Geometry check sheet. Reference: the model listing, model coordinates, mm. A direction names the side the tool comes from. Coordinates: 2 decimals unless noted, no trailing zeros. Loops run counter-clockwise (first coordinate to the right, second up) from the corner with the lowest first, then second, coordinate; pieces in that order, holes last.
Autodesk Inventor part; units mm, degrees
ref_plane "Work Plane1" through (0, -20.15, 0) normal (-1, 0, 0) x (0, 0, 1)
ref_plane "YZ Plane" through (0, 0, 0) normal (1, 0, 0) x (0, 1, 0)
ref_plane "XZ Plane" through (0, 0, 0) normal (0, 1, 0) x (-1, 0, 0)
sketch "Sketch1" plane through (0, 0, 0) normal (0, 0, 1) x (1, 0, 0)
  line L0 (-12.05, 27.5) -> (12.05, 27.5)
  line L1 (12.05, 27.5) -> (12.05, -27.5)
  line L2 (12.05, -27.5) -> (-12.05, -27.5)
  line L3 (-12.05, -27.5) -> (-12.05, 27.5)
  line L4 (-10.05, 20.15) -> (10.05, 20.15)
  line L5 (10.05, 20.15) -> (10.05, -20.15)
  line L6 (10.05, -20.15) -> (-10.05, -20.15)
  line L7 (-10.05, -20.15) -> (-10.05, 20.15)
  line L8 (0, 0) -> (0, 17.7516) construction
  line L9 (0, 0) -> (17.0454, 0) construction
  line L10 (-12.05, -27.5) -> (12.05, -27.5)
  line L11 (12.05, -27.5) -> (12.05, -20.15)
  line L12 (12.05, -20.15) -> (-12.05, -20.15)
  line L13 (-12.05, -20.15) -> (-12.05, -27.5)
  circle A0 centre (-4.65, 24.5) radius 2.175
  circle A1 centre (4.65, 24.475) radius 2.175
  circle A2 centre (-4.6492, -24.5) radius 2.175
  circle A3 centre (4.65, -24.375) radius 2.175
  point P0 (12.05, -23.825)
  dimension "d0" = 40.3
  dimension "d1" = 20.1
  dimension "d2" = 55
  dimension "d3" = 24.1
  dimension "d4" = 4.35
  dimension "d5" = 4.325
  dimension "d6" = 4.35
  dimension "d8" = 4.35
  dimension "d9" = 5.4
  dimension "d13" = 5.4
  dimension "d28" = 48.85
  dimension "d29" = 9.3
  dimension "d30" = 9.3
extrude "Extrusion1" add sketch "Sketch1" along normal blind 5 contours L0 L1 L12 L5 L4 L7 L3 | L12 L6 L1 L2 L3
extrude "Extrusion2" add sketch "Sketch1" against normal blind 15 contours L12 L6 L1 L2 L3 | A2 | A3
extrude "Extrusion3" cut sketch "Sketch1" against normal blind 3 contours A2 | A3
sketch "Sketch2" plane through (-10.05, -20.15, 5) normal (0, 1, 0) x (1, 0, 0)
  circle A0 centre (5.9, 16) radius 1.05
  circle A1 centre (14.2, 16) radius 1.05
  line L0 (0, 0) -> (20.1, 0) construction
  line L1 (10.05, 0) -> (10.05, 23.167) construction
  line L2 (-2, 20) -> (22.1, 20)
  circle A2 centre (14.2, 16) radius 2
  circle A3 centre (5.9, 16) radius 2
  point P0 (10.05, 5)
  dimension "d20" = 2.1
  dimension "d21" = 8.3
  dimension "d22" = 4
  dimension "d23" = 4
extrude "Extrusion4" cut sketch "Sketch2" against normal blind 10 contours A0 | A1
extrude "Extrusion5" cut sketch "Sketch2" against normal blind 3 contours A0 | A1 | A2 | A3
sketch "Sketch3" plane through (12.05, -20.15, 0) normal (1, 0, 0) x (0, 0, -1)
  line L0 (0, 47.65) -> (-5, 47.65) construction
  line L1 (-5, 47.65) -> (38.6712, 47.65) construction
  line L2 (0, 0) -> (-5, 0) construction
  line L3 (-5, 0) -> (38.6712, 0) construction
  line L4 (0, 15) -> (15, 0)
  line L5 (0, 15) -> (0, 9.3431)
  line L6 (0, 9.3431) -> (9.3431, 0)
  line L7 (9.3431, 0) -> (15, 0)
  line L8 (15, 0) -> (15, -7.35) construction
  line L9 (15, -0.9137) -> (15, 2.4866) construction
  line L10 (-5, 0) -> (15, 0)
  line L11 (15, 0) -> (15, -15)
  line L12 (15, -15) -> (-5, -15)
  line L13 (-5, -15) -> (-5, 0)
  circle A0 centre (5, -12.35) radius 1.25
  line L14 (0, 0) -> (0, 47.65)
  line L15 (0, 47.65) -> (0, 0)
  line L16 (0, 0) -> (15, 0)
  line L17 (15, -7.35) -> (15, 0)
  line L18 (15, -7.35) -> (-5, -7.35)
  line L19 (-5, 47.65) -> (-5, -7.35)
  line L20 (0, 47.65) -> (-5, 47.65)
  point P0 (0, 20.15)
  dimension "d31" = 4
  dimension "d34" = 15
  dimension "d39" = 2.5
  dimension "d41" = 10
  dimension "d44" = 45
  dimension "d46" = 5
ref_plane "Work Plane1" through (0, -20.15, 0) normal (-1, 0, 0) x (0, 0, 1)
extrude "Extrusion6" add sketch "Sketch3" against normal up to surface (2 mm away) contours L4 L7 L6 L5
mirror "Mirror1" about plane through (0, -20.15, 0) normal (-1, 0, 0) of "Extrusion6"
extrude "Extrusion7" add sketch "Sketch3" along normal blind 3.9 from surface at -24.1 contours L11 L18 L13 L10 L7 | L11 L12 L13 L18 | A0
extrude "Extrusion8" cut sketch "Sketch3" against normal blind 35.65 contours A0
equation "\"d8\" = d6"
equation "\"d13\" = d9"
properties part number "BIGServoHolder"
1) Material ranges on probe 1 along X at (y, z) = (-21.8, -11); probe 2 along X at (y, z) = (-25.85, -11); probe 3 along Y at (x, z) = (4.65, 2), recorded low to high.
Data:
probe 1: x = -12.05 to -6.15, -2.15 to 2.15, 6.15 to 12.05
probe 2: x = -12.05 to -5.2, -3.1 to 3.1, 5.2 to 12.05
probe 3: y = -27.5 to -26.55, -22.2 to -20.15, 20.15 to 22.3, 26.65 to 27.5
2) Access from +Z, -Z, +X, -X, +Y, -Y to the whole of each face (thin tool, end or side, straight path). Record for faces 4 (the flat face through (2, -27.5, -5)), 5 (the flat face through (-11.064, -15.544, -4.737)), 6 (the flat face through (0, 20.15, 2)).
Data:
face 4: +Z, -Z, +X, -Y
face 5: +X, -X
face 6: +Z, -Z
3) Section check C-C on x = 4.15. Record the cut outline in (y, z).
Data:
outline: (-27.5, -15) - (-20.15, -15) - (-20.15, -13) - (-23.15, -13) - (-23.15, -12.05) - (-27.5, -12.05) - close; (-27.5, -9.95) - (-23.15, -9.95) - (-23.15, -9) - (-20.15, -9) - (-20.15, 5) - (-22.26, 5) - (-22.26, -3) - (-26.49, -3) - (-26.49, 5) - (-27.5, 5) - close; (20.15, 0) - (22.36, 0) - (22.36, 5) - (20.15, 5) - close; (26.59, 0) - (27.5, 0) - (27.5, 5) - (26.59, 5) - close
4) Mould release check, pull along X, two halves, no side actions. Record for faces 1 (the cylindrical face through (-10.073, -33.609, -5.577)), 2 (the flat face through (-8.15, -30, -5)), 3 (the flat face through (-3, -23.15, -10)): +X half, -X half, draft (parallel to the pull), parting line (faces both ways), or undercut.
Data:
face 1: draft
face 2: +X half
face 3: undercut
5) Depth check by flat-ended pin: pin 1 (2.5 mm diameter, centred on x = 4.15, z = -11, fed in from -Y); pin 2 (3 mm diameter, centred on x = -4.15, z = -11, fed in from +Y); pin 3 (1 mm diameter, centred on x = 10.5, y = -16.5, fed in from -Z). Enter the tip coordinate at first touch or a pass-through.
Data:
pin 1: stops at y = -27.5
pin 2: stops at y = -23.15
pin 3: stops at z = -11.85
6) Section check A-A on z = -11. Record the cut outline in (x, y).
Data:
outline: (-12.05, -35.15) - (-8.15, -35.15) - (-8.15, -27.5) - (-5.2, -27.5) - (-5.2, -23.15) - (-6.15, -23.15) - (-6.15, -20.15) - (-10.05, -20.15) - (-10.05, -16.15) - (-12.05, -16.15) - close; (-3.1, -27.5) - (3.1, -27.5) - (3.1, -23.15) - (2.15, -23.15) - (2.15, -20.15) - (-2.15, -20.15) - (-2.15, -23.15) - (-3.1, -23.15) - close; (5.2, -27.5) - (12.05, -27.5) - (12.05, -16.15) - (10.05, -16.15) - (10.05, -20.15) - (6.15, -20.15) - (6.15, -23.15) - (5.2, -23.15) - close
7) Section check D-D on z = -1.25. Record the cut outline in (x, y) (3 decimals).
Data:
outline: (-12.05, -35.15) - (-8.15, -35.15) - (-8.15, -27.5) - (12.05, -27.5) - (12.05, -20.15) - (-12.05, -20.15) - close; (-12.05, -12.057) - (-10.05, -12.057) - (-10.05, -6.4) - (-12.05, -6.4) - close; (10.05, -12.057) - (12.05, -12.057) - (12.05, -6.4) - (10.05, -6.4) - close; hole circle Ø4.35 at (-4.649, -24.5); hole circle Ø4.35 at (4.65, -24.375)
8) Section check B-B on y = -32.5. Record the cut outline in (x, z), and give its area (4 significant figures).
Data:
outline: (-12.05, -15) - (-8.15, -15) - (-8.15, -6.25) - (-12.05, -6.25) - close; (-12.05, -3.75) - (-8.15, -3.75) - (-8.15, 5) - (-12.05, 5) - close
area: 68.25 mm2
